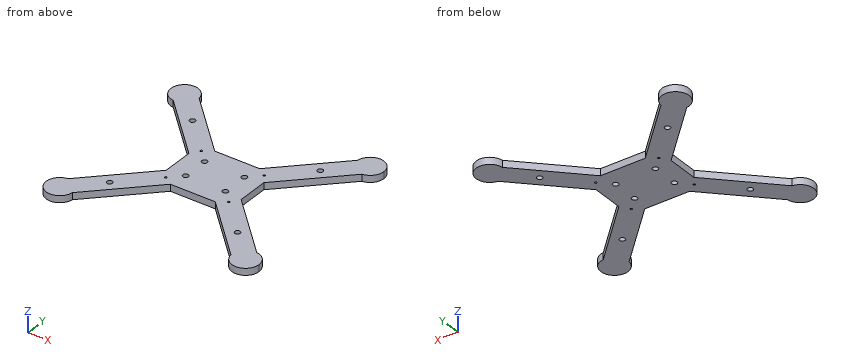
```python
from build123d import *

# Parameters (mm, degrees)
ESQUISSE1_W             = 110
ESQUISSE1_H             = 90
BOSS_EXTRU_1_DEPTH      = 10
ESQUISSE3_R             = 4
ESQUISSE3_R_2           = 1.6
ENL_V_MAT_EXTRU_2_DEPTH = 215.345138396


with BuildPart() as part:
    # Esquisse1 → Boss.-Extru.1 (new body)
    with BuildSketch(Plane.XY):
        with BuildLine():
            ThreePointArc((-116.429085419, 128.429085419), (-150.45941546, 140.45941546), (-138.429085419, 106.429085419))
            Line((-138.429085419, 106.429085419), (-147.317279836, 115.317279836))
            Line((-147.317279836, 115.317279836), (-125.317279836, 137.317279836))
            Line((-125.317279836, 137.317279836), (-116.429085419, 128.429085419))
        make_face()
        with BuildLine():
            Line((-147.317279836, 115.317279836), (-138.429085419, 106.429085419))
            ThreePointArc((-138.429085419, 106.429085419), (-122.942604357, 111.447240972), (-116.317279836, 126.317279836))
            ThreePointArc((-116.317279836, 126.317279836), (-116.345250791, 127.374661426), (-116.429085419, 128.429085419))
            Line((-116.429085419, 128.429085419), (-125.317279836, 137.317279836))
            Line((-125.317279836, 137.317279836), (-147.317279836, 115.317279836))
        make_face()
        with BuildLine():
            Line((-138.429085419, 106.429085419), (-55, 23))
            Line((-55, 23), (-55, 45))
            Line((-55, 45), (-33, 45))
            Line((-33, 45), (-116.429085419, 128.429085419))
            ThreePointArc((-116.429085419, 128.429085419), (-116.345250791, 127.374661426), (-116.317279836, 126.317279836))
            ThreePointArc((-116.317279836, 126.317279836), (-122.942604357, 111.447240972), (-138.429085419, 106.429085419))
        make_face()
        with BuildLine():
            Line((116.429085419, 128.429085419), (33, 45))
            Line((33, 45), (55, 45))
            Line((55, 45), (55, 23))
            Line((55, 23), (138.429085419, 106.429085419))
            ThreePointArc((138.429085419, 106.429085419), (122.175144213, 112.175144213), (116.429085419, 128.429085419))
        make_face()
        with BuildLine():
            ThreePointArc((156.317279836, 126.317279836), (137.374661426, 146.289308881), (116.429085419, 128.429085419))
            Line((116.429085419, 128.429085419), (125.317279836, 137.317279836))
            Line((125.317279836, 137.317279836), (147.317279836, 115.317279836))
            Line((147.317279836, 115.317279836), (138.429085419, 106.429085419))
            ThreePointArc((138.429085419, 106.429085419), (151.187318701, 112.942604357), (156.317279836, 126.317279836))
        make_face()
        with BuildLine():
            Line((125.317279836, 137.317279836), (116.429085419, 128.429085419))
            ThreePointArc((116.429085419, 128.429085419), (122.175144213, 112.175144213), (138.429085419, 106.429085419))
            Line((138.429085419, 106.429085419), (147.317279836, 115.317279836))
            Line((147.317279836, 115.317279836), (125.317279836, 137.317279836))
        make_face()
        Rectangle(ESQUISSE1_W, ESQUISSE1_H)
        with BuildLine():
            ThreePointArc((138.429085419, -106.429085419), (122.175144213, -112.175144213), (116.429085419, -128.429085419))
            Line((116.429085419, -128.429085419), (125.317279836, -137.317279836))
            Line((125.317279836, -137.317279836), (147.317279836, -115.317279836))
            Line((147.317279836, -115.317279836), (138.429085419, -106.429085419))
        make_face()
        with BuildLine():
            Line((125.317279836, -137.317279836), (116.429085419, -128.429085419))
            ThreePointArc((116.429085419, -128.429085419), (137.374661426, -146.289308881), (156.317279836, -126.317279836))
            ThreePointArc((156.317279836, -126.317279836), (151.187318701, -112.942604357), (138.429085419, -106.429085419))
            Line((138.429085419, -106.429085419), (147.317279836, -115.317279836))
            Line((147.317279836, -115.317279836), (125.317279836, -137.317279836))
        make_face()
        with BuildLine():
            Line((55, -45), (33, -45))
            Line((33, -45), (116.429085419, -128.429085419))
            ThreePointArc((116.429085419, -128.429085419), (122.175144213, -112.175144213), (138.429085419, -106.429085419))
            Line((138.429085419, -106.429085419), (55, -23))
            Line((55, -23), (55, -45))
        make_face()
        with BuildLine():
            ThreePointArc((-116.317279836, -126.317279836), (-122.942604357, -111.447240972), (-138.429085419, -106.429085419))
            Line((-138.429085419, -106.429085419), (-147.317279836, -115.317279836))
            Line((-147.317279836, -115.317279836), (-125.317279836, -137.317279836))
            Line((-125.317279836, -137.317279836), (-116.429085419, -128.429085419))
            ThreePointArc((-116.429085419, -128.429085419), (-116.345250791, -127.374661426), (-116.317279836, -126.317279836))
        make_face()
        with BuildLine():
            Line((-147.317279836, -115.317279836), (-138.429085419, -106.429085419))
            ThreePointArc((-138.429085419, -106.429085419), (-150.45941546, -140.45941546), (-116.429085419, -128.429085419))
            Line((-116.429085419, -128.429085419), (-125.317279836, -137.317279836))
            Line((-125.317279836, -137.317279836), (-147.317279836, -115.317279836))
        make_face()
        with BuildLine():
            Line((-55, -45), (-55, -23))
            Line((-55, -23), (-138.429085419, -106.429085419))
            ThreePointArc((-138.429085419, -106.429085419), (-122.942604357, -111.447240972), (-116.317279836, -126.317279836))
            ThreePointArc((-116.317279836, -126.317279836), (-116.345250791, -127.374661426), (-116.429085419, -128.429085419))
            Line((-116.429085419, -128.429085419), (-33, -45))
            Line((-33, -45), (-55, -45))
        make_face()
    extrude(amount=BOSS_EXTRU_1_DEPTH)

    # Esquisse3 → Enlèv. mat.-Extru.2 (cut, through all)
    with BuildSketch(Plane(origin=(0, 0, 0), x_dir=(-1, 0, 0), z_dir=(0, 0, -1))):
        with Locations(Location((93.890872965, 83.890872965, 0), (0, 0, 180))):
            Circle(ESQUISSE3_R)
        with Locations((-93.890872965, 83.890872965)):
            Circle(ESQUISSE3_R)
        with Locations((-29.238399287, 19.238399287)):
            Circle(ESQUISSE3_R)
        with Locations((-46, 36)):
            Circle(ESQUISSE3_R_2)
        with Locations((46, 36)):
            Circle(ESQUISSE3_R_2)
        with Locations((46, -36)):
            Circle(ESQUISSE3_R_2)
        with Locations((-46, -36)):
            Circle(ESQUISSE3_R_2)
        with Locations(Location((29.238399287, 19.238399287, 0), (0, 0, 180))):
            Circle(ESQUISSE3_R)
        with Locations(Location((-93.890872965, -83.890872965, 0), (0, 0, 180))):
            Circle(ESQUISSE3_R)
        with Locations(Location((-29.238399287, -19.238399287, 0), (0, 0, 180))):
            Circle(ESQUISSE3_R)
        with Locations((29.238399287, -19.238399287)):
            Circle(ESQUISSE3_R)
        with Locations((93.890872965, -83.890872965)):
            Circle(ESQUISSE3_R)
    extrude(amount=-ENL_V_MAT_EXTRU_2_DEPTH, mode=Mode.SUBTRACT)


solid = part.part
```
CAD build for the part. Positions are in the model's coordinates, mm. Coordinates: 2 decimals unless noted, no trailing zeros. Order: outer loops, then holes, each group sorted by start corner. A loop starts at its lowest first (then second) coordinate and runs counter-clockwise, first axis right, second up.
(1) Pin check, flat tips, straight feed: pin 1 Ø1.5 at (y, z) = (37, 1.5) entering from +X; pin 2 Ø7 at (x, y) = (29.24, -19.24) entering from -Z; pin 3 Ø1.5 at (y, z) = (-10, 2.5) entering from -X; pin 4 Ø3 at (x, z) = (-7, 5.5) entering from +Y. Stop position of each tip, or through.
Solution:
pin 1: stops at x = 69.75
pin 2: passes through
pin 3: stops at x = -55
pin 4: stops at y = 45
(2) Saw through at B-B, the plane y = 54. Write the cut outline in (x, z), and give its area (3 significant figures).
Solution:
outline: (-86, 0) - (-42, 0) - (-42, 10) - (-86, 10) - close; (42, 0) - (86, 0) - (86, 10) - (42, 10) - close
area: 880 mm2
(3) Saw through at D-D, the plane x = 10. Write the cut outline in (y, z), and give its area (3 significant figures).
Solution:
outline: (-45, 0) - (45, 0) - (45, 10) - (-45, 10) - close
area: 900 mm2
(4) Saw through at C-C, the plane z = 3.5. Count the separate pieces of the cut face and the enclosed holes in it, and give its area (3 significant figures).
Solution:
separate pieces: 1
enclosed holes: 12
area: 27,600 mm2
(5) Saw through at A-A, the plane x = 75.5. Write the cut outline in (y, z), and give its area (3 significant figures).
Solution:
outline: (-87.5, 0) - (-43.5, 0) - (-43.5, 10) - (-87.5, 10) - close; (43.5, 0) - (87.5, 0) - (87.5, 10) - (43.5, 10) - close
area: 880 mm2
(6) Drill centre lines: L1, parallel to Y at x = 46, z = 4.75; L2, parallel to Y at x = 92, z = 8.25; L3, parallel to Y at x = 7.5, z = 6.25. Where is each one in solid material? Low to high.
Solution:
L1: y = -58 to -37.6, -34.4 to 34.4, 37.6 to 58
L2: y = -104 to -87.42, -80.37 to -60, 60 to 80.37, 87.42 to 104
L3: y = -45 to 45
